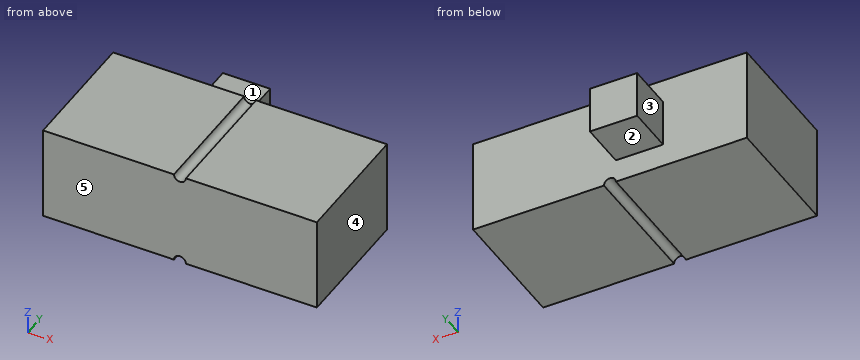
```python
from build123d import *

# Parameters (mm, degrees)
SKETCH1_W               = 11.6
SKETCH1_H               = 5.4102
BOSS_EXTRUDE1_DEPTH     = 4
SKETCH2_W               = 2
SKETCH2_H               = 2
BOSS_EXTRUDE2_DEPTH     = 2
CUT_EXTRUDE1_DEPTH      = 9.883144941
CUT_EXTRUDE1_DEPTH_BACK = 9.883144941


with BuildPart() as part:
    # Sketch1 → Boss-Extrude1 (new body)
    with BuildSketch(Plane.XY):
        Rectangle(SKETCH1_W, SKETCH1_H)
    extrude(amount=BOSS_EXTRUDE1_DEPTH)

    # Sketch2 → Boss-Extrude2 (add)
    with BuildSketch(Plane(origin=(0, 2.7051, 0), x_dir=(1, 0, 0), z_dir=(0, 1, 0))):
        with Locations((-1.25, -2)):
            Rectangle(SKETCH2_W, SKETCH2_H)
    extrude(amount=BOSS_EXTRUDE2_DEPTH)

    # Sketch3 → Cut-Extrude1 (cut, two sides: drawn at the far end of the back side and taken through both)
    with BuildSketch(Plane(origin=(0, 2.7051, 0), x_dir=(1, 0, 0), z_dir=(0, 1, 0)).offset(-CUT_EXTRUDE1_DEPTH_BACK)):
        with BuildLine():
            Line((-0.254, 0), (0.254, 0))
            ThreePointArc((0.254, 0), (0, -0.254), (-0.254, 0))
        make_face()
        with BuildLine():
            Line((-0.254, -4), (0.254, -4))
            ThreePointArc((0.254, -4), (0, -3.746), (-0.254, -4))
        make_face()
    extrude(amount=CUT_EXTRUDE1_DEPTH + CUT_EXTRUDE1_DEPTH_BACK, mode=Mode.SUBTRACT)


solid = part.part
```
Input: part model. Units: mm. Frame: model coordinates. Face numbers are marked on the shaded views. A direction names the side the tool comes from. Round coordinates to 2 decimals unless told otherwise and drop trailing zeros. Order: outer loops, then holes, each group sorted by start corner. A loop starts at its lowest first (then second) coordinate and runs counter-clockwise, first axis right, second up. Notation, with made-up numbers: (3, 54) - (10, 54) arc R26 cw to (10, 79) - close; hole circle Ø3 at (-14.75, 22.5). An arc over 180 degrees is marked (long way). Answer in a Markdown table with one row per item.
Item 1: Line query: line 1 (Y direction, x = 2.25, z = 0.7); line 2 (X direction, y = 4.25, z = 1.85); line 3 (Z direction, x = -1, y = 3). Output: solid intervals per line, ascending.
Model answer:
| item | result |
|---|---|
| line 1 | y = -2.71 to 2.71 |
| line 2 | x = -2.25 to -0.25 |
| line 3 | z = 1 to 3 |
Item 2: Section query B-B (x = -0.75). Return the cut outline in (y, z).
Model answer:
| item | result |
|---|---|
| outline | (-2.71, 0) - (2.71, 0) - (2.71, 1) - (4.71, 1) - (4.71, 3) - (2.71, 3) - (2.71, 4) - (-2.71, 4) - close |
Item 3: Section query A-A (z = 1.75). Return the cut outline in (x, y).
Model answer:
| item | result |
|---|---|
| outline | (-5.8, -2.71) - (5.8, -2.71) - (5.8, 2.71) - (-0.25, 2.71) - (-0.25, 4.71) - (-2.25, 4.71) - (-2.25, 2.71) - (-5.8, 2.71) - close |
Item 4: Reachability of the marked faces 1, 2, 3, 4 and 5 from +Z, -Z, +X, -X, +Y, -Y: full face, straight path, thin tool, end or side. Return the list, or none.
Model answer:
| item | result |
|---|---|
| face 1 | +Z, +X, -X, +Y |
| face 2 | -Z, +X, -X, +Y |
| face 3 | +Z, -Z, -X, +Y |
| face 4 | +Z, -Z, +X, +Y, -Y |
| face 5 | +Z, -Z, +X, -X, -Y |
Item 5: Section query D-D (z = 0.45). Return the cut outline in (x, y), then the cut area to 3 significant figures.
Model answer:
| item | result |
|---|---|
| outline | (-5.8, -2.71) - (5.8, -2.71) - (5.8, 2.71) - (-5.8, 2.71) - close |
| area | 62.8 mm² |
Item 6: Pin query (flat end, axial travel): pin 1 (0.6 mm diameter, centred on y = 3.5, z = 1.5, fed in from -X); pin 2 (1.6 mm diameter, centred on x = -1, y = 4, fed in from -Z). Return the tip coordinate at first contact, or that it passes through.
Model answer:
| item | result |
|---|---|
| pin 1 | stops at x = -2.25 |
| pin 2 | stops at z = 1 |
Item 7: Section query C-C (x = -3). Return the cut outline in (y, z), then the cut area to 3 significant figures.
Model answer:
| item | result |
|---|---|
| outline | (-2.71, 0) - (2.71, 0) - (2.71, 4) - (-2.71, 4) - close |
| area | 21.6 mm² |
